The listing builds one solid part. Answer for the finished solid, in the listing's coordinates (mm). Give positions to 0.01 mm unless a question says otherwise; leave off trailing zeros. Write each loop counter-clockwise with the first axis right and the second up, starting at its lowest first coordinate (ties: lowest second). Pieces come first, ordered by that corner, then holes. Notation, with made-up numbers: (36, -14.75) - (56, -14.75) arc R24 cw to (56, 20.25) - close; hole circle Ø1 at (-38, 65.25). An arc over 180 degrees is marked (long way). Use a Markdown table: item, result. Add a question column.
from build123d import *

# Parameters (mm, degrees)
SKETCH1_R           = 3.951125178
SKETCH1_R_2         = 3.606945722
SKETCH1_R_3         = 3.375000002
SKETCH1_R_4         = 3.375000001
SKETCH1_R_5         = 3.374999999
BOSS_EXTRUDE1_DEPTH = 6


with BuildPart() as part:
    # Sketch1 → Boss-Extrude1 (new body)
    with BuildSketch(Plane(origin=(0, 0, 0), x_dir=(1, 0, 0), z_dir=(0, 1, 0))):
        Polygon((-41.199524293, 99.465227688), (99.465250609, 99.465227688), (99.465250609, -99.465227688), (-41.199524293, -99.465227688), (-99.465227688, -41.199524293), (-99.465227688, 41.199524293), align=None)
        with Locations((0, -86.090250609)):
            Circle(SKETCH1_R, mode=Mode.SUBTRACT)
        with Locations((-86.090250609, 0)):
            Circle(SKETCH1_R_2, mode=Mode.SUBTRACT)
        with Locations((-60.875, 60.875)):
            Circle(SKETCH1_R_2, mode=Mode.SUBTRACT)
        with Locations((0, 86.090250609)):
            Circle(SKETCH1_R_2, mode=Mode.SUBTRACT)
        with Locations((60.875, 60.875)):
            Circle(SKETCH1_R_2, mode=Mode.SUBTRACT)
        with Locations((86.090250609, 0)):
            Circle(SKETCH1_R_2, mode=Mode.SUBTRACT)
        with Locations((60.875, -60.875)):
            Circle(SKETCH1_R_2, mode=Mode.SUBTRACT)
        with Locations((-60.875, -60.875)):
            Circle(SKETCH1_R_2, mode=Mode.SUBTRACT)
        with Locations((80.004750061, -86.090249939)):
            Circle(SKETCH1_R_3, mode=Mode.SUBTRACT)
        with Locations((-6.085500548, 6.7e-07)):
            Circle(SKETCH1_R_4, mode=Mode.SUBTRACT)
        with Locations((80.004750061, 86.09025128)):
            Circle(SKETCH1_R_5, mode=Mode.SUBTRACT)
    extrude(amount=BOSS_EXTRUDE1_DEPTH)


solid = part.part
1. The part is cut by section A-A (x = 0). Give the vertices of the cut face in (y, z).
2. For a pull along X with two mould halves and no side action, classify faces 1 (the cylindrical face through (-9.457, 2.958, -0.148)), 2 (the flat face through (30, 3, 99.465)), 3 (the flat face through (99.465, 3, -1)) as released by +X, released by -X, zero draft, split by the parting line, or undercut.
3. Given P1, Ø6.5, axis at x = -60.875, z = 60.875, coming from the -Y side, flat-ended and moving along its own axis, determine where the tip first touches the part or whether it passes through.
4. Consider L1, parallel to X at y = 2.25, z = 0; L2, parallel to Z at x = 0, y = 2.35; L3, parallel to X at y = 0.5, z = 0.5. Determine where each line is inside the solid, lowest interval first. Write a range as [from, to].
5. The part is cut by section B-B (z = 0). Give the vertices of the cut face in (x, y).
6. The part is cut by section C-C (y = 3). Count the separate pieces of the cut face and the enclosed holes in it, and give its area (3 significant figures).
7. The part is cut by section D-D (z = 51). Give the vertices of the cut face in (x, y).
Check values:
| question | item | result |
|---|---|---|
| 1 | outline | (0, -99.47) - (6, -99.47) - (6, -89.7) - (0, -89.7) - close; (0, -82.48) - (6, -82.48) - (6, 82.14) - (0, 82.14) - close; (0, 90.04) - (6, 90.04) - (6, 99.47) - (0, 99.47) - close |
| 2 | face 1 | undercut |
| 2 | face 2 | zero draft |
| 2 | face 3 | released by +X |
| 3 | P1 | passes through |
| 4 | L1 | x = [-99.47, -89.7], [-82.48, -9.46], [-2.71, 82.48], [89.7, 99.47] |
| 4 | L2 | z = [-99.47, -89.7], [-82.48, 82.14], [90.04, 99.47] |
| 4 | L3 | x = [-99.47, -89.66], [-82.52, -9.42], [-2.75, 82.52], [89.66, 99.47] |
| 5 | outline | (-99.47, 0) - (-89.7, 0) - (-89.7, 6) - (-99.47, 6) - close; (-82.48, 0) - (-9.46, 0) - (-9.46, 6) - (-82.48, 6) - close; (-2.71, 0) - (82.48, 0) - (82.48, 6) - (-2.71, 6) - close; (89.7, 0) - (99.47, 0) - (99.47, 6) - (89.7, 6) - close |
| 6 | separate pieces | 1 |
| 6 | enclosed holes | 11 |
| 6 | area | 35,700 mm2 |
| 7 | outline | (-89.66, 0) - (99.47, 0) - (99.47, 6) - (-89.66, 6) - close |
